```python
from build123d import *

# Parameters (mm, degrees)
SKETCH1_R           = 40
BOSS_EXTRUDE1_DEPTH = 16
SKETCH2_W           = 41
SKETCH2_H           = 41
CUT_EXTRUDE1_DEPTH  = 59.787753827
BOSS_EXTRUDE2_DEPTH = 5
BOSS_EXTRUDE3_DEPTH = 5


with BuildPart() as part:
    # Sketch1 → Boss-Extrude1 (new body)
    with BuildSketch(Plane(origin=(0, 0, 0), x_dir=(1, 0, 0), z_dir=(0, 1, 0))):
        with Locations(Location((0, 0, 0), (0, 0, 270))):
            Circle(SKETCH1_R)
    extrude(amount=BOSS_EXTRUDE1_DEPTH)

    # Sketch2 → Cut-Extrude1 (cut, through all)
    with BuildSketch(Plane(origin=(0, 16, 0), x_dir=(1, 0, 0), z_dir=(0, 1, 0))):
        Rectangle(SKETCH2_W, SKETCH2_H)
    extrude(amount=-CUT_EXTRUDE1_DEPTH, mode=Mode.SUBTRACT)

    # Sweep1: sweep along a path in Sketch10
    with BuildLine(Plane(origin=(0, 16, 0), x_dir=(1, 0, 0), z_dir=(0, 1, 0))) as sweep1_path:
        ThreePointArc((-20, -34.641016151), (0, -40), (20, -34.641016151))
    # Sketch3 → Sweep1 (sweep)
    with BuildSketch(Plane.ZY):
        with BuildLine():
            Line((40, 0), (40, 16))
            Line((40, 16), (40, 31.584891677))
            Line((40, 31.584891677), (45, 31.584891677))
            ThreePointArc((45, 31.584891677), (92.852664778, -46.723418702), (184.367988058, -39.866698948))
            Line((184.367988058, -39.866698948), (187.286623743, -43.926448415))
            ThreePointArc((187.286623743, -43.926448415), (105.473564082, -57.24807138), (45.527749442, 0))
            Line((45.527749442, 0), (40, 0))
        make_face()
    sweep(path=sweep1_path.line)

    # Sketch11 → Boss-Extrude2 (add)
    with BuildSketch(Plane(origin=(0, 0, 0), x_dir=(-0.5000000000000012, 0, -0.8660254037844378), z_dir=(0.8660254037844379, 0, -0.5000000000000013))):
        with BuildLine():
            Line((-184.367988058, -39.866698948), (-179.698170962, -33.3710998))
            ThreePointArc((-179.698170962, -33.3710998), (-96.502422525, -39.604481395), (-53, 31.584891677))
            Line((-53, 31.584891677), (-45, 31.584891677))
            Line((-45, 31.584891677), (-40, 31.584891677))
            Line((-40, 31.584891677), (-40, 16))
            Line((-40, 16), (-40, 0))
            Line((-40, 0), (-45.527749442, 0))
            ThreePointArc((-45.527749442, 0), (-105.473564082, -57.24807138), (-187.286623743, -43.926448415))
            Line((-187.286623743, -43.926448415), (-184.367988058, -39.866698948))
        make_face()
    extrude(amount=BOSS_EXTRUDE2_DEPTH)

    # Sketch12 → Boss-Extrude3 (add)
    with BuildSketch(Plane(origin=(0, 0, 0), x_dir=(-0.5000000000000012, 0, 0.866025403784438), z_dir=(-0.866025403784438, 0, -0.5000000000000012))):
        with BuildLine():
            Line((45, 31.584891677), (53, 31.584891677))
            ThreePointArc((53, 31.584891677), (96.502422525, -39.604481395), (179.698170962, -33.3710998))
            Line((179.698170962, -33.3710998), (184.367988058, -39.866698948))
            Line((184.367988058, -39.866698948), (187.286623743, -43.926448415))
            ThreePointArc((187.286623743, -43.926448415), (105.473564082, -57.24807138), (45.527749442, 0))
            Line((45.527749442, 0), (40, 0))
            Line((40, 0), (40, 16))
            Line((40, 16), (40, 31.584891677))
            Line((40, 31.584891677), (45, 31.584891677))
        make_face()
    extrude(amount=BOSS_EXTRUDE3_DEPTH)


solid = part.part
```
Could you check a few things on this model? Use its own coordinates, in mm. A direction names the side the tool comes from. Round coordinates to 2 decimals unless told otherwise and drop trailing zeros. Loops run counter-clockwise (first coordinate to the right, second up) from the corner with the lowest first, then second, coordinate; pieces in that order, holes last. Notation, with made-up numbers: M 63,-37 L 108,-37 A10 cw 108,-31 Z; hole C -6.75,35 d7. An arc over 180 degrees is marked long. Answer as CSV lines item,"result".
1) Imagine slicing it at D-D on y = -10. List the corners of the cut face in (x, z) for me.
From the geometry:
outline,"M -36.66,53.5 L -29.24,40.64 L -24.91,43.14 A49.82 cw 24.91,43.14 L 29.24,40.64 L 36.66,53.5 L 32.33,56 L 27.72,48.02 A55.45 ccw -27.72,48.02 L -32.33,56 Z"
2) If I drill on probe 1 along Z at (x, y) = (44, -45.5); probe 2 along Y at (x, z) = (-29.5, 1); probe 3 along Z at (x, y) = (-17, 5.5), over which ranges is the centre line in solid material (lowest first)?
From the geometry:
probe 1,"68.09 to 79.14, 169.84 to 179.72"
probe 2,"0 to 16"
probe 3,"-36.21 to -20.5, 20.5 to 45.91"
3) Imagine slicing it at B-B on z = 0. List the corners of the cut face in (x, y) for me, and give its area (3 significant figures).
From the geometry:
outline,"M -40,0 L -20.5,0 L -20.5,16 L -40,16 Z; M 20.5,0 L 40,0 L 40,16 L 20.5,16 Z"
area,"624 mm^2"
4) Which directions (+Z, -Z, +X, -X, +Y, -Y) give clear straight access to the entire face, cutting with the end or side of a thin tool? Please do faces 1 (the flat face through (-49.76, -41.54, 86.19)), 2 (the flat face through (1, 16, 26)), 3 (the cylindrical face through (54.298, -56.885, 89.117)), 4 (the flat face through (0, 8, -20.5)).
From the geometry:
face 1,"+Y"
face 2,"-Z, +Y"
face 3,"-Y"
face 4,"+Y, -Y"
5) Imagine slicing it at A-A on x = 0. List the corners of the cut face in (y, z) for me.
From the geometry:
outline,"M -43.93,187.29 A93 ccw 0,45.53 L 0,20.5 L 16,20.5 L 16,40 L 31.58,40 L 31.58,45 A88 cw -39.87,184.37 Z; M 0,-40 L 16,-40 L 16,-20.5 L 0,-20.5 Z"
6) Imagine slicing it at C-C on y = 3.5. List the corners of the cut face in (x, z) for me.
From the geometry:
outline,"M -33.38,47.81 L -24.33,32.14 L -20,34.64 A40 ccw long 20,34.64 L 24.33,32.14 L 33.38,47.81 L 29.05,50.31 L 24.8,42.96 A49.6 ccw -24.8,42.96 L -29.05,50.31 Z; hole M -20.5,-20.5 L 20.5,-20.5 L 20.5,20.5 L -20.5,20.5 Z"
7) For pin 1 Ø5 at (y, z) = (8, 12.5) entering from +X; pin 2 Ø24 at (x, z) = (19, -11.5) entering from -Y; pin 3 Ø13 at (y, z) = (9.5, -7) entering from +X, each with a flat end and sliding along its axis, tell me the tip position at first contact or that it passes through.
From the geometry:
pin 1,"x = 38.73"
pin 2,"y = 0"
pin 3,"x = 40"
8) We'd pull the mould along X, two halves only. Please class faces 5 (the flat face through (-50.413, -38.809, 77.319)), 6 (the flat face through (0, 8, 20.5)), 7 (the flat face through (50.07, -38.81, 76.72)): released by +X, released by -X, zero draft, split by the parting line, or undercut.
From the geometry:
face 5,"released by -X"
face 6,"undercut"
face 7,"released by +X"
